Can you work these out from the model? Positions are in its coordinate system, mm. A direction names the side the tool comes from. Coordinates: 2 decimals unless noted, no trailing zeros. Write each loop counter-clockwise with the first axis right and the second up, starting at its lowest first coordinate (ties: lowest second). Pieces come first, ordered by that corner, then holes. Notation, with made-up numbers: (76, 32.5) - (96, 32.5) arc R5 cw to (96, 39.5) - close; hole circle Ø11 at (26.5, 45.5). An arc over 180 degrees is marked (long way). One line per question, with ' | ' between items. Start each with the question number.
from build123d import *

# Parameters (mm, degrees)
SKETCH1_R               = 10.3632
BOSS_EXTRUDE1_DEPTH     = 15.875
BOSS_EXTRUDE2_DEPTH     = 5.842
SKETCH3_R               = 3.131421561
BOSS_EXTRUDE3_DEPTH     = 3.175
BOSS_EXTRUDE4_DEPTH     = 12.573
SKETCH5_R               = 10.4775
BOSS_EXTRUDE5_DEPTH     = 6.2865
SKETCH6_R               = 6.63575
BOSS_EXTRUDE6_DEPTH     = 10.795
SKETCH7_R               = 9.525
BOSS_EXTRUDE7_DEPTH     = 9.525
SKETCH9_R               = 8.7376
BOSS_EXTRUDE8_DEPTH     = 0.79375
SKETCH10_R              = 9.525
BOSS_EXTRUDE9_DEPTH     = 12.7
CUT_EXTRUDE1_DEPTH      = 1.5875
CUT_EXTRUDE2_REACH      = 51.292
CUT_EXTRUDE2_END_RADIUS = 9.525
SKETCH12_W              = 3.175
SKETCH12_H              = 3.175
BOSS_EXTRUDE10_DEPTH    = 6.35
SKETCH13_W              = 1.5875
SKETCH13_H              = 3.175
BOSS_EXTRUDE11_DEPTH    = 12.7
BOSS_EXTRUDE12_DEPTH    = 3.175
BOSS_EXTRUDE13_DEPTH    = 3.175
SKETCH17_W              = 1.953483497
SKETCH17_H              = 9.525
BOSS_EXTRUDE14_DEPTH    = 1.5875
CUT_EXTRUDE3_REACH      = 50.413
SKETCH21_R              = 2.667
SKETCH22_R              = 2.54
CUT_EXTRUDE4_DEPTH      = 27.94


with BuildPart() as part:
    # Sketch1 → Boss-Extrude1 (new body)
    with BuildSketch(Plane(origin=(0, 0, 0), x_dir=(0, 0, -1), z_dir=(1, 0, 0))):
        Circle(SKETCH1_R)
    extrude(amount=-BOSS_EXTRUDE1_DEPTH)

    # Sketch2 → Boss-Extrude2 (add)
    with BuildSketch(Plane.ZY.offset(15.875)):
        Polygon((6.397302804, 11.106241349), (-6.419635747, 11.093347418), (-12.81693855, -0.012893931), (-6.397302804, -11.106241349), (6.419635747, -11.093347418), (12.81693855, 0.012893931), align=None)
    extrude(amount=BOSS_EXTRUDE2_DEPTH)

    # Sketch3 → Boss-Extrude3 (add)
    with BuildSketch(Plane.ZY.offset(21.717)):
        Circle(SKETCH3_R)
    extrude(amount=BOSS_EXTRUDE3_DEPTH)

    # Sketch4 → Boss-Extrude4 (add)
    with BuildSketch(Plane.ZY.offset(24.892)):
        Polygon((-12.648301022, 0), (-6.324150511, -10.95375), (6.324150511, -10.95375), (12.648301022, 0), (6.324150511, 10.95375), (-6.324150511, 10.95375), align=None)
    extrude(amount=BOSS_EXTRUDE4_DEPTH)

    # Sketch5 → Boss-Extrude5 (add)
    with BuildSketch(Plane.ZY.offset(37.465)):
        Circle(SKETCH5_R)
    extrude(amount=BOSS_EXTRUDE5_DEPTH)

    # Sketch6 → Boss-Extrude6 (add)
    with BuildSketch(Plane(origin=(0, 0, 0), x_dir=(0, 0, -1), z_dir=(1, 0, 0))):
        Circle(SKETCH6_R)
    extrude(amount=BOSS_EXTRUDE6_DEPTH)

    # Sketch7 → Boss-Extrude7 (add)
    with BuildSketch(Plane(origin=(10.795, 0, 0), x_dir=(0, 0, -1), z_dir=(1, 0, 0))):
        with Locations(Location((0, 0, 0), (0, 0, 180))):
            Circle(SKETCH7_R)
    extrude(amount=BOSS_EXTRUDE7_DEPTH)

    # Sketch9 → Boss-Extrude8 (add)
    with BuildSketch(Plane(origin=(20.32, 0, 0), x_dir=(0, 0, -1), z_dir=(1, 0, 0))):
        Circle(SKETCH9_R)
    extrude(amount=BOSS_EXTRUDE8_DEPTH)

    # Sketch10 → Boss-Extrude9 (add)
    with BuildSketch(Plane(origin=(21.11375, 0, 0), x_dir=(0, 0, -1), z_dir=(1, 0, 0))):
        with Locations(Location((0, 0, 0), (0, 0, 180))):
            Circle(SKETCH10_R)
    extrude(amount=BOSS_EXTRUDE9_DEPTH)

    # Sketch11 → Cut-Extrude1 (cut)
    with BuildSketch(Plane.XY.offset(-6.985)):
        Polygon((27.46375, 5.844282471), (27.46375, -5.844282471), (20.32, -5.844282471), (20.32, -1.410545514), (23.495, -1.410545514), (23.495, 1.410545514), (20.32, 1.410545514), (20.32, 5.844282471), align=None)
    extrude(amount=CUT_EXTRUDE1_DEPTH, mode=Mode.SUBTRACT)

    # Cut-Extrude2: up to this cylinder (the profile starts inside it)
    cut_extrude2_end = Plane(origin=(24.130314, 0, 0), z_dir=(-1, 0, 0)) * Cylinder(CUT_EXTRUDE2_END_RADIUS, 122.634, mode=Mode.PRIVATE)
    # Sketch11<2> → Cut-Extrude2 (cut, up to the surface)
    with BuildSketch(Plane.XY.offset(-6.985), mode=Mode.PRIVATE) as cut_extrude2_sk1:
        Polygon((27.46375, 5.844282471), (27.46375, -5.844282471), (20.32, -5.844282471), (20.32, -1.410545514), (23.495, -1.410545514), (23.495, 1.410545514), (20.32, 1.410545514), (20.32, 5.844282471), align=None)
    cut_extrude2_tool1 = extrude(cut_extrude2_sk1.sketch, amount=-CUT_EXTRUDE2_REACH, mode=Mode.PRIVATE) & cut_extrude2_end
    add(cut_extrude2_tool1.solids().sort_by_distance((24.130314, 0, -6.985))[0], mode=Mode.SUBTRACT)

    # Sketch12 → Boss-Extrude10 (add)
    with BuildSketch(Plane(origin=(0, 0, -5.3975), x_dir=(-1, 0, 0), z_dir=(0, 0, -1))):
        with Locations((-24.69818991, -3.175)):
            Rectangle(SKETCH12_W, SKETCH12_H)
        with Locations((-24.69818991, 3.175)):
            Rectangle(SKETCH12_W, SKETCH12_H)
    extrude(amount=BOSS_EXTRUDE10_DEPTH)

    # Sketch13 → Boss-Extrude11 (add)
    with BuildSketch(Plane.ZY.offset(-23.11068991)):
        with Locations((-10.95375, -3.175)):
            Rectangle(SKETCH13_W, SKETCH13_H)
        with Locations((-10.95375, 3.175)):
            Rectangle(SKETCH13_W, SKETCH13_H)
    extrude(amount=BOSS_EXTRUDE11_DEPTH)

    # Sketch14 → Boss-Extrude12 (add)
    with BuildSketch(Plane.XZ.offset(4.7625)):
        Polygon((12.364173407, -10.16), (10.141014473, -13.335), (8.187530976, -13.335), (10.41068991, -10.16), align=None)
    extrude(amount=-BOSS_EXTRUDE12_DEPTH)

    # Sketch16 → Boss-Extrude13 (add)
    with BuildSketch(Plane(origin=(0, 4.7625, 0), x_dir=(1, 0, 0), z_dir=(0, 1, 0))):
        Polygon((10.41068991, 10.16), (8.187530976, 13.335), (10.141014473, 13.335), (12.364173407, 10.16), align=None)
    extrude(amount=-BOSS_EXTRUDE13_DEPTH)

    # Sketch17 → Boss-Extrude14 (add)
    with BuildSketch(Plane(origin=(0, 0, -13.335), x_dir=(-1, 0, 0), z_dir=(0, 0, -1))):
        with Locations((-9.164272724, 0)):
            Rectangle(SKETCH17_W, SKETCH17_H)
    extrude(amount=-BOSS_EXTRUDE14_DEPTH)

    # Sketch18 → Cut-Extrude3 (cut, up to next)
    with BuildSketch(Plane(origin=(0, 4.7625, 0), x_dir=(1, 0, 0), z_dir=(0, 1, 0)), mode=Mode.PRIVATE) as cut_extrude3_sk1:
        Polygon((10.41068991, 10.16), (8.187530976, 13.335), (8.187530976, 10.16), align=None)
    cut_extrude3_tool1 = extrude(cut_extrude3_sk1.sketch, amount=-CUT_EXTRUDE3_REACH, mode=Mode.PRIVATE) & part.part
    add(cut_extrude3_tool1.solids().sort_by_distance((8.928584, 4.7625, -11.218333))[0], mode=Mode.SUBTRACT)

    # Sweep1: sweep along a path in Sketch19
    with BuildLine(Plane(origin=(0, 0, 0), x_dir=(1, 0, 0), z_dir=(0, 1, 0))) as sweep1_path:
        Line((33.81375, 0), (84.61375, 0))
        ThreePointArc((84.61375, 0), (135.41375, -50.8), (84.61375, -101.6))
        Line((84.61375, -101.6), (0, -101.6))
    # Sketch21 → Sweep1 (sweep)
    with BuildSketch(Plane(origin=(0, 0, 0), x_dir=(0, 0, -1), z_dir=(1, 0, 0))):
        with Locations((-101.6, 0)):
            Circle(SKETCH21_R)
    sweep(path=sweep1_path.line)

    # Sketch22 → Cut-Extrude4 (cut)
    with BuildSketch(Plane.ZY.offset(43.7515)):
        Circle(SKETCH22_R)
    extrude(amount=-CUT_EXTRUDE4_DEPTH, mode=Mode.SUBTRACT)


solid = part.part
(1) If I drill on probe 1 along Y at (x, z) = (-28, 0); probe 2 along Y at (x, z) = (-37.75, 0); probe 3 along Y at (x, z) = (32.5, -7), over which ranges is the centre line in solid material (lowest first)?
(2) If we section it at A-A on x = 58: List the corners of the cut face in (y, z) for me, plus the area to 3 significant figures.
(3) If we mould it in two halves opening along X, with no side actions, what happens to faces 5 (the face through (-40.56, 10.39, -1.36)), 6 (the face through (-24.892, 3, 3)), 7 (the face through (-43.752, -2, 2))? For each: +X half, -X half, draft (parallel to the pull), parting line (faces both ways), or undercut.
(4) Which directions (+Z, -Z, +X, -X, +Y, -Y) give clear straight access to the entire face, cutting with the end or side of a thin tool? Please do faces 1 (the face through (27.464, 0, -7)), 2 (the face through (-15.875, -1.6, 10.4)), 3 (the face through (-15.811, 0, 0)), 4 (the face through (-18.755, 5.618, -9.574)).
(5) I'm going to push flat-ended pins straight in: pin 1 (2.5 mm diameter, centred on y = 1.5, z = 102, fed in from -X); pin 2 (10 mm diameter, centred on x = 96, y = -3, fed in from -Z); pin 3 (4 mm diameter, centred on x = 105.5, y = 2.5, fed in from +Z). Where does each tip first touch, or does it pass through?
Values:
1) probe 1: -10.95 to -2.54, 2.54 to 10.95 | probe 2: -10.48 to -2.54, 2.54 to 10.48 | probe 3: -6.46 to 6.46
2) outline: circle Ø5.33 at (0, 0); circle Ø5.33 at (0, 101.6) | area: 44.7 mm2
3) face 5: draft | face 6: undercut | face 7: -X half
4) face 1: -Z | face 2: none | face 3: -X | face 4: -Z, -X, +Y
5) pin 1: x = 0 | pin 2: z = -2.17 | pin 3: z = 100.35
